Design review of the part shown in the three views and the two pictorial views. Dimensions are in mm from the part's minimum x, y and z. A direction names the side the tool comes from. Round coordinates to 2 decimals unless told otherwise and drop trailing zeros. Order: outer loops, then holes, each group sorted by start corner. A loop starts at its lowest first (then second) coordinate and runs counter-clockwise, first axis right, second up. Notation, with made-up numbers: M 77.25,4.5 L 134.25,4.5 A13 ccw 134.25,20.5 Z; hole C 80,4 d9. An arc over 180 degrees is marked long. Write each question's results on one line, items separated by ' | '. Start each with the question number.
Item 1: The part is to be moulded in two halves that separate along Y. For the marked faces 3, 4, 5 and 6, say which applies: +Y half, -Y half, draft (parallel to the pull), parting line (faces both ways), or undercut.
Item 2: Machinability: for the marked faces 1 and 2, which of the approach directions +Z, -Z, +X, -X, +Y, -Y give a long, thin tool a straight path to every point of the face, cutting with its end or side? Answer none if there is none.
Item 3: Take a section at C-C, the plane z = 1. Write out the cut boundary in (x, y).
Item 4: Take a section at A-A, the plane y = 37. Write out the cut boundary in (x, z).
Item 5: Take a section at D-D, the plane z = 5. Write out the cut boundary in (x, y).
Item 6: Take a section at B-B, the plane x = 50. Write out the cut boundary in (y, z).
Item 7: Clearance check with a flat-ended pin moving along its axis: pin 1 (4 mm diameter, centred on x = 53.5, z = 5, fed in from +Y). State where the tip first meets the part, or that it passes through.
Item 8: Wall thickness on line 1 (Y direction, x = 50, z = 7); line 2 (Y direction, x = 37, z = 4.75); line 3 (X direction, y = 6, z = 7): over which ranges is each line inside the solid? List them lowest first. Write a range as [from, to].
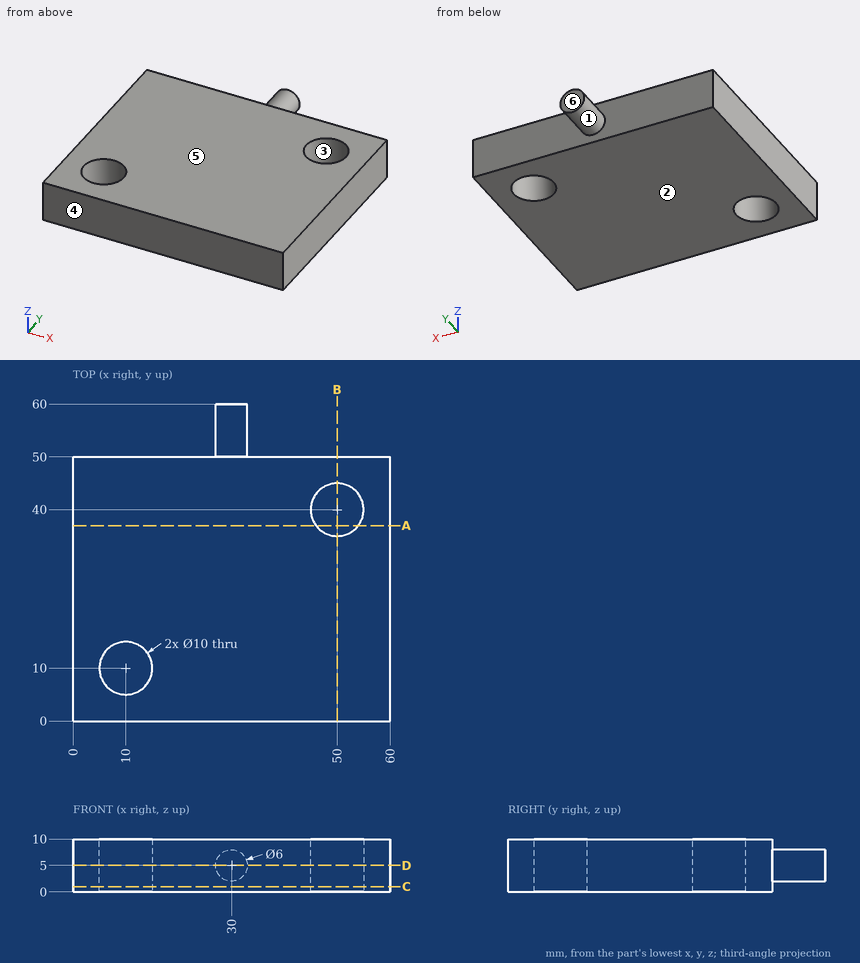
Results list:
1) face 3: undercut | face 4: -Y half | face 5: draft | face 6: +Y half
2) face 1: +Y | face 2: -Z, +X, -X, +Y, -Y
3) outline: M 0,0 L 60,0 L 60,50 L 0,50 Z; hole C 10,10 d10; hole C 50,40 d10
4) outline: M 0,0 L 46,0 L 46,10 L 0,10 Z; M 54,0 L 60,0 L 60,10 L 54,10 Z
5) outline: M 0,0 L 60,0 L 60,50 L 33,50 L 33,60 L 27,60 L 27,50 L 0,50 Z; hole C 10,10 d10; hole C 50,40 d10
6) outline: M 0,0 L 35,0 L 35,10 L 0,10 Z; M 45,0 L 50,0 L 50,10 L 45,10 Z
7) pin 1: y = 50
8) line 1: [0, 35], [45, 50] | line 2: [0, 50] | line 3: [0, 7], [13, 60]
